Autodesk Inventor part; units mm, degrees
ref_plane "Angled_top_face" through (-52.5, 25, 47.5) normal (0, -0.819152, -0.5735764) x (1, 0, 0)
ref_plane "YZ Plane" through (0, 0, 0) normal (1, 0, 0) x (0, 1, 0)
ref_plane "XZ Plane" through (0, 0, 0) normal (0, 1, 0) x (-1, 0, 0)
sketch "XZ_master" plane through (0, 0, 0) normal (0, 1, 0) x (-1, 0, 0)
  line L0 (52.5, -47.5) -> (-52.5, -47.5)
  line L1 (-52.5, -47.5) -> (-52.5, 47.5)
  line L2 (-52.5, 47.5) -> (52.5, 47.5)
  line L3 (52.5, 47.5) -> (52.5, -47.5)
  line L4 (52.5, -47.5) -> (-52.5, 47.5) construction
  line L5 (-52.5, -47.5) -> (52.5, 47.5) construction
  line L6 (50.5, -45.5) -> (-50.5, -45.5)
  line L7 (-50.5, -45.5) -> (-50.5, 45.5)
  line L8 (-50.5, 45.5) -> (50.5, 45.5)
  line L9 (50.5, 45.5) -> (50.5, -45.5)
  point P0 (0, 0)
  dimension "d0" = 105
  dimension "d1" = 95
  dimension "d2" = 2
sketch "XZ_master outline for Walls_bottom" plane through (0, 0, 0) normal (0, 1, 0) x (-1, 0, 0)
  line L0 (52.5, -47.5) -> (52.5, 47.5)
  line L1 (-52.5, -47.5) -> (52.5, -47.5)
  line L2 (52.5, 47.5) -> (-52.5, 47.5)
  line L3 (-52.5, 47.5) -> (-52.5, -47.5)
  line L4 (50.5, -45.5) -> (-50.5, -45.5)
  line L5 (50.5, 45.5) -> (50.5, -45.5)
  line L6 (-50.5, 45.5) -> (50.5, 45.5)
  line L7 (-50.5, -45.5) -> (-50.5, 45.5)
extrude "Walls_bottom" add sketch "XZ_master outline for Walls_bottom" along normal blind 25
fillet "Fillet2" radius 0.75 4 edges at (0, 0, 45.5) (50.5, 0, 0) (-50.5, 0, 0) (0, 0, -45.5)
sketch "Profile" plane through (0, 0, 0) normal (1, 0, 0) x (0, 1, 0)
  line L0 (0, 45.5) -> (25, 45.5)
  line L1 (2, 45.5) -> (4, 45.5)
  line L2 (4, 45.5) -> (4, 46.7)
  line L3 (4, 46.7) -> (2, 46.7)
  line L4 (2, 46.7) -> (2, 45.5)
  line L5 (0, -47.5) -> (0, 47.5)
  circle A0 centre (10.654636, -35.042492) radius 3.75
  line L6 (4, 46.7) -> (4, -38.2) construction
  line L7 (4, 46.7) -> (88.9, 46.7) construction
  point P0 (0, 0)
  dimension "d5" = 2
  dimension "d6" = 1.2
  dimension "d7" = 2
  dimension "d27" = 7.5
  dimension "d30" = 90
sketch "Profile outline for Lip recess" plane through (0, 0, 0) normal (1, 0, 0) x (0, 1, 0)
  line L0 (4, 46.7) -> (2, 46.7)
  line L1 (4, 45.5) -> (4, 46.7)
  line L2 (2, 45.5) -> (4, 45.5)
  line L3 (2, 46.7) -> (2, 45.5)
extrude "Lip recess" cut sketch "Profile outline for Lip recess" along normal mid plane 101
fillet "Lip_fillet" radius 1 2 edges at (0, 4, 45.5) (0, 2, 45.5)
pattern_circular "Circular Pattern1" count 2 over 360 about axis through (0, -10, 0) along (0, 1, 0) of "Lip recess"
ref_plane "Angled_top_face" through (-52.5, 25, 47.5) normal (0, -0.819152, -0.5735764) x (1, 0, 0)
sketch "XZ_master outline for Walls_to_workplane" plane through (0, 0, 0) normal (0, 1, 0) x (-1, 0, 0)
  line L0 (52.5, -47.5) -> (52.5, 47.5)
  line L1 (-52.5, -47.5) -> (52.5, -47.5)
  line L2 (52.5, 47.5) -> (-52.5, 47.5)
  line L3 (-52.5, 47.5) -> (-52.5, -47.5)
  line L4 (50.5, -45.5) -> (-50.5, -45.5)
  line L5 (50.5, 45.5) -> (50.5, -45.5)
  line L6 (-50.5, 45.5) -> (50.5, 45.5)
  line L7 (-50.5, -45.5) -> (-50.5, 45.5)
extrude "Walls_to_workplane" add sketch "XZ_master outline for Walls_to_workplane" along normal up to surface from surface at 25 surface through (-52.5, 25, 47.5) normal (0, -0.819152, -0.5735764)
sketch "Top_face" plane through (-52.5, 25, 47.5) normal (0, -0.819152, -0.5735764) x (1, 0, 0)
  line L0 (105, -115.973586) -> (0, -115.973586)
  line L1 (0, 0) -> (105, 0)
  line L2 (105, 0) -> (105, -115.973586)
  line L3 (105, -115.973586) -> (0, -115.973586)
  line L4 (0, -115.973586) -> (0, 0)
  line L5 (0, -115.973586) -> (0, 0) construction
  line L6 (2, -2.441549) -> (2, -113.532037)
  line L7 (2, -113.532037) -> (103, -113.532037)
  line L8 (103, -113.532037) -> (103, -2.441549)
  line L9 (103, -2.441549) -> (2, -2.441549)
  line L10 (105, 0) -> (105, -115.973586)
  line L11 (105, -115.973586) -> (0, -115.973586)
  line L12 (0, -115.973586) -> (0, 0)
  line L13 (0, 0) -> (105, 0)
  line L14 (2, -113.532037) -> (103, -113.532037) construction
  line L15 (52.5, -113.532037) -> (52.5, -2.441549) construction
  line L16 (103, -2.441549) -> (2, -2.441549) construction
  circle A0 centre (52.5, -53.441549) radius 44
  circle A1 centre (52.5, -97.441549) radius 3
  circle A2 centre (52.5, -9.441549) radius 3
  circle A3 centre (52.5, -53.441549) radius 46
  circle A4 centre (52.5, -97.441549) radius 5
  circle A5 centre (52.5, -9.441549) radius 5
  circle A6 centre (52.5, -53.441549) radius 13.5
  circle A7 centre (52.5, -53.441549) radius 51 construction
  point P0 (55.498256, -97.339276)
  point P1 (55.498256, -9.543822)
  point P2 (49.501744, -9.543822)
  point P3 (49.501744, -97.339276)
  point P4 (47.820513, -99.202913)
  point P5 (57.179487, -99.202913)
  point P6 (57.179487, -7.680186)
  point P7 (47.820513, -7.680186)
  dimension "d61" = 88
  dimension "d62" = 51
  dimension "d63" = 6
  dimension "d64" = 6
  dimension "d65" = 2
  dimension "d66" = 2
  dimension "d67" = 2
  dimension "d68" = 27
  dimension "d69" = 102
sketch "Top_face outline for Face" plane through (-52.5, 25, 47.5) normal (0, -0.819152, -0.5735764) x (1, 0, 0)
  line L0 (105, -115.973586) -> (105, 0)
  line L1 (0, -115.973586) -> (105, -115.973586)
  line L2 (0, 0) -> (0, -115.973586)
  line L3 (105, 0) -> (0, 0)
extrude "Face" add sketch "Top_face outline for Face" against normal blind 2 draft -35
sketch "Top_face outline for Button_recess" plane through (-52.5, 25, 47.5) normal (0, -0.819152, -0.5735764) x (1, 0, 0)
  arc A0 (49.501744, -97.339276) -> (55.498256, -97.339276) centre (52.5, -97.441549) ccw
  arc A1 (49.501744, -9.543822) -> (49.501744, -97.339276) centre (52.5, -53.441549) ccw
  arc A2 (55.498256, -9.543822) -> (49.501744, -9.543822) centre (52.5, -9.441549) ccw
  arc A3 (55.498256, -97.339276) -> (55.498256, -9.543822) centre (52.5, -53.441549) ccw
extrude "Button_recess" cut sketch "Top_face outline for Button_recess" against normal through all draft 15
sketch "Profile outline for Side_cable_cutout" plane through (0, 0, 0) normal (1, 0, 0) x (0, 1, 0)
  circle A0 centre (10.654636, -35.042492) radius 3.75
extrude "Side_cable_cutout" cut sketch "Profile outline for Side_cable_cutout" against normal through all
sketch "Top_face outline for Recess_walls" plane through (-52.5, 25, 47.5) normal (0, -0.819152, -0.5735764) x (1, 0, 0)
  arc A0 (47.820513, -99.202913) -> (57.179487, -99.202913) centre (52.5, -97.441549) ccw
  arc A1 (47.820513, -7.680186) -> (47.820513, -99.202913) centre (52.5, -53.441549) ccw
  arc A2 (57.179487, -99.202913) -> (57.179487, -7.680186) centre (52.5, -53.441549) ccw
  arc A3 (57.179487, -7.680186) -> (47.820513, -7.680186) centre (52.5, -9.441549) ccw
  arc A4 (55.498256, -97.339276) -> (49.501744, -97.339276) centre (52.5, -97.441549) cw
  arc A5 (55.498256, -9.543822) -> (55.498256, -97.339276) centre (52.5, -53.441549) cw
  arc A6 (49.501744, -9.543822) -> (55.498256, -9.543822) centre (52.5, -9.441549) cw
  arc A7 (49.501744, -97.339276) -> (49.501744, -9.543822) centre (52.5, -53.441549) cw
extrude "Recess_walls" add sketch "Top_face outline for Recess_walls" along normal blind 8.5
sketch "Top_face outline for Recess_floor" plane through (-52.5, 25, 47.5) normal (0, -0.819152, -0.5735764) x (1, 0, 0)
  arc A0 (47.820513, -99.202913) -> (57.179487, -99.202913) centre (52.5, -97.441549) ccw
  arc A1 (47.820513, -7.680186) -> (47.820513, -99.202913) centre (52.5, -53.441549) ccw
  arc A2 (57.179487, -99.202913) -> (57.179487, -7.680186) centre (52.5, -53.441549) ccw
  arc A3 (57.179487, -7.680186) -> (47.820513, -7.680186) centre (52.5, -9.441549) ccw
  circle A4 centre (52.5, -53.441549) radius 13.5
extrude "Recess_floor" add sketch "Top_face outline for Recess_floor" along normal blind 2 from surface at 8.5
chamfer "Button_cutout_chamfer" distance 1 angle 45 1 edges at (-13.5, 48.69, -1.1522)
properties part number "BARB_top" material "ABS Plastic"
Read the model definition and answer for the solid it produces. Units are mm, in the model's axes. A direction names the side the tool comes from. Give positions to 0.01 mm unless a question says otherwise; leave off trailing zeros. Order: outer loops, then holes, each group sorted by start corner. A loop starts at its lowest first (then second) coordinate and runs counter-clockwise, first axis right, second up.
(1) Find section A-A (y = 16). Give the vertices of the cut face in (x, z), plus the area to 3 significant figures.
(2) For a pull along Y with two mould halves and no side action, classify faces 1 (the flat face through (52.5, 35, -10)), 2 (the cylindrical face through (45.99, 50.87, 1.53)), 3 (the flat face through (-51.81, 58.6, 1.23)), 4 (the cylindrical face through (0.08, 79.52, -39.38)) as released by +Y, released by -Y, zero draft, split by the parting line, or undercut.
(3) Straight lines are drawn through the part: L1, parallel to Z at x = 17.5, y = 22; L2, parallel to X at y = 61, z = -39; L3, parallel to Z at x = 25.5, y = 26. For each, find the intervals that lie inside material, in ascending order.
(4) Given pin 1 (1.3 mm diameter, centred on x = 22, z = -46.5, fed in from +Y); pin 2 (8 mm diameter, centred on x = -39.5, z = 2.5, fed in from +Y); pin 3 (1 mm diameter, centred on x = -18.5, z = -15, fed in from +Y), each flat-ended and moving along its own axis, determine where each tip first touches the part or whether it passes through.
(5) For faces 5 (the cylindrical face through (-51.486, 9.842, -38.703)), 6 (the conical face through (-44.083, 56.469, 3.163)), 7 (the flat face through (-52.5, 35, -11)), 8 (the flat face through (1, 16, 45.5)), determine the directions among +Z, -Z, +X, -X, +Y, -Y from which every point of the face is accessible in a straight line to the end or side of a thin tool.
Result sheet:
1. outline: (-52.5, -47.5) - (52.5, -47.5) - (52.5, 47.5) - (-52.5, 47.5) - close; hole (-50.5, -45.5) - (50.5, -45.5) - (50.5, 45.5) - (-50.5, 45.5) - close
1. area: 784 mm2
2. face 1: zero draft
2. face 2: undercut
2. face 3: released by +Y
2. face 4: undercut
3. L1: z = -47.5 to -45.5, 45.5 to 47.5
3. L2: x = -52.5 to -50.5, 50.5 to 52.5
3. L3: z = -47.5 to -45.5, 27.77 to 29.7, 45.5 to 47.5
4. pin 1: stops at y = 92.12
4. pin 2: stops at y = 48.93
4. pin 3: stops at y = 58.74
5. face 5: -X
5. face 6: none
5. face 7: +Z, -Z, -X, +Y, -Y
5. face 8: -Y
